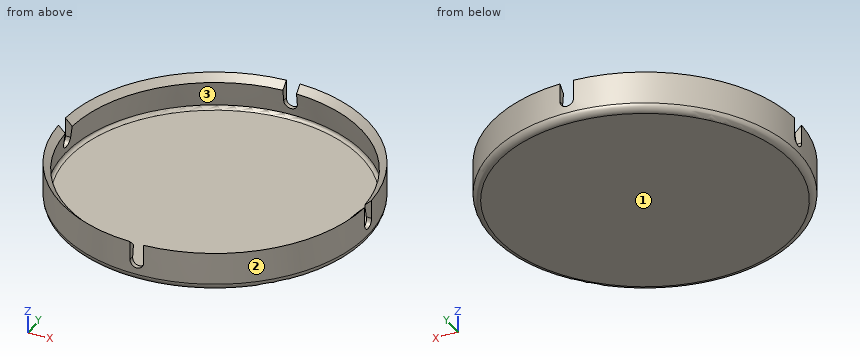
from build123d import *

# Parameters (mm, degrees)
F3_DEPTH = 50
F5_DEPTH = 50


with BuildPart() as f1:
    # F0 (on Front) → F1 (revolve)
    with BuildSketch(Plane.XZ):
        with BuildLine():
            Line((-43, 9.5), (-45, 11.5))
            Line((-45, 11.5), (-45, 2))
            ThreePointArc((-45, 2), (-44.414214, 0.585786), (-43, 0))
            Line((-43, 0), (0, 0))
            Line((0, 0), (0, 1))
            Line((0, 1), (-43, 1))
            ThreePointArc((-43, 1), (-43.707107, 1.292893), (-44, 2))
            Line((-44, 2), (-43, 9.5))
        make_face()
    revolve(axis=Axis((0, 0, 0.5), (0, 0, -1)))

    # F2 (on Front) → F3 (cut, symmetric)
    with BuildSketch(Plane.XZ):
        with BuildLine():
            Line((-2, 11.5), (-2, 6))
            ThreePointArc((-2, 6), (0, 4), (2, 6))
            Line((2, 6), (2, 11.5))
            Line((2, 11.5), (-2, 11.5))
        make_face()
    extrude(amount=F3_DEPTH, both=True, mode=Mode.SUBTRACT)

    # F4 (on Right) → F5 (cut, symmetric)
    with BuildSketch(Plane.YZ):
        with BuildLine():
            Line((-2, 11.5), (-2, 6))
            ThreePointArc((-2, 6), (0, 4), (2, 6))
            Line((2, 6), (2, 11.5))
            Line((2, 11.5), (-2, 11.5))
        make_face()
    extrude(amount=F5_DEPTH, both=True, mode=Mode.SUBTRACT)


solid = f1.part
For this review, take the finished solid that the model builds, in its own axes (mm). Face numbers are marked on the shaded views. Round coordinates to 2 decimals unless told otherwise and drop trailing zeros. Loops run counter-clockwise (first coordinate to the right, second up) from the corner with the lowest first, then second, coordinate; pieces in that order, holes last. Notation, with made-up numbers: (83.5, -3.75) - (126.5, -3.75) arc R19 cw to (126.5, 22.25) - close; hole circle Ø10 at (6.5, 11). An arc over 180 degrees is marked (long way). Answer as CSV lines item,"result".
(1) Mouldability with a two-part tool opening along Y and no side actions: class the marked faces 1, 2 and 3 as +Y half, -Y half, draft (parallel to the pull), parting line (faces both ways), or undercut.
Checked values:
face 1,"draft"
face 2,"parting line"
face 3,"undercut"
(2) Wall thickness on line 1 (Z direction, x = -35, y = 21); line 2 (Y direction, x = 14, z = 10); line 3 (X direction, y = -2.5, z = 4): over which ranges is each line inside the solid? List them lowest first.
Checked values:
line 1,"z = 0 to 1"
line 2,"y = -42.77 to -41.19, 41.19 to 42.77"
line 3,"x = -44.93 to -43.66, 43.66 to 44.93"
(3) Insertion check: P1, Ø3, axis at x = -2, y = -7.5, coming from the +Z side; P2, Ø3, axis at x = 29, z = 7, coming from the +Y side; P3, Ø1, axis at x = -17.5, z = 7.5, coming from the -Y side. Each pin has a flat end and moves straight along its axis. Give the tip position at first contact, or say it passes through.
Checked values:
P1,"stops at z = 1"
P2,"stops at y = 35.62"
P3,"stops at y = -41.67"
(4) Consider section B-B on x = 0. Give the boundary of the cut face in (y, z).
Checked values:
outline,"(-45, 2) arc R2 ccw to (-43, 0) - (43, 0) arc R2 ccw to (45, 2) - (45, 4) - (43.73, 4) - (44, 2) arc R1 cw to (43, 1) - (-43, 1) arc R1 cw to (-44, 2) - (-43.73, 4) - (-45, 4) - close"
